Could you check a few things on this model? Use its own coordinates, in mm. Face numbers are marked on the shaded views. A direction names the side the tool comes from. Give positions to 0.01 mm unless a question says otherwise; leave off trailing zeros. Order: outer loops, then holes, each group sorted by start corner. A loop starts at its lowest first (then second) coordinate and runs counter-clockwise, first axis right, second up. Notation, with made-up numbers: (10, 27) -> (15, 27) arc R10 ccw to (15, 34) -> close; hole circle Ø6 at (37.25, 57). An arc over 180 degrees is marked (long way). One line per item, written item: value.
```python
from build123d import *

# Parameters (mm, degrees)
SKETCH1_W           = 55
SKETCH1_H           = 38
SKETCH1_R           = 14.2875
BOSS_EXTRUDE3_DEPTH = 8
SKETCH8_W           = 6
SKETCH8_H           = 38
BOSS_EXTRUDE6_DEPTH = 35
FILLET1_R           = 1
SKETCH9_R           = 2.5
CUT_EXTRUDE1_DEPTH  = 10


with BuildPart() as part:
    # Sketch1 → Boss-Extrude3 (new body)
    with BuildSketch(Plane.XY):
        with Locations((27.5, 19)):
            Rectangle(SKETCH1_W, SKETCH1_H)
        with Locations((35, 19)):
            Circle(SKETCH1_R, mode=Mode.SUBTRACT)
    extrude(amount=BOSS_EXTRUDE3_DEPTH)

    # Sketch8 → Boss-Extrude6 (add)
    with BuildSketch(Plane(origin=(0, 0, 0), x_dir=(-1, 0, 0), z_dir=(0, 0, -1))):
        with Locations((-3, 19)):
            Rectangle(SKETCH8_W, SKETCH8_H)
    extrude(amount=BOSS_EXTRUDE6_DEPTH)

    # Fillet1
    fillet1_edges = [part.edges().sort_by_distance(p)[0] for p in [
        (6, 19, 0),
    ]]
    fillet(fillet1_edges, radius=FILLET1_R)

    # Sketch9 → Cut-Extrude1 (cut)
    with BuildSketch(Plane(origin=(6, 0, 0), x_dir=(0, 0, -1), z_dir=(1, 0, 0))):
        with Locations((8.157894737, 30)):
            Circle(SKETCH9_R)
        with Locations((8.157894737, 8)):
            Circle(SKETCH9_R)
        with Locations((27.842105263, 8)):
            Circle(SKETCH9_R)
        with Locations((27.842105263, 30)):
            Circle(SKETCH9_R)
    extrude(amount=-CUT_EXTRUDE1_DEPTH, mode=Mode.SUBTRACT)


solid = part.part
```
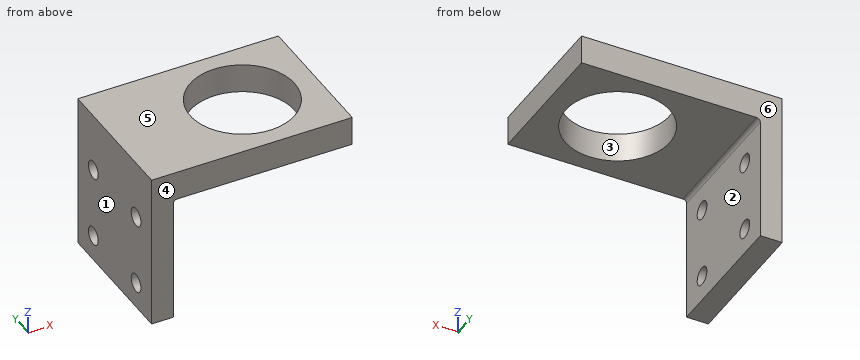
1) If I drill on line 1 along X through (y, z) = (18.5, 4.5); line 2 along Y through (x, z) = (35, 2); line 3 along Z through (x, y) = (52.5, 16), over which ranges is the centre line in solid material (lowest first)?
Answer below:
line 1: x = 0 to 20.72, 49.28 to 55
line 2: y = 0 to 4.71, 33.29 to 38
line 3: z = 0 to 8
2) Suppose I cut it at D-D, the plane y = 3.5. Write out the boundary of the cut face in (x, z).
Answer below:
outline: (0, -35) -> (6, -35) -> (6, -1) arc R1 cw to (7, 0) -> (55, 0) -> (55, 8) -> (0, 8) -> close
3) For P1, Ø2, axis at y = 6.5, z = -27.5, coming from the +X side; P2, Ø6, axis at x = 14.5, y = 19.5, coming from the -Z side; P3, Ø4, axis at y = 30, z = -27.84, coming from the -X side, each with a flat end and sliding along its axis, tell me the tip position at first contact or that it passes through.
Answer below:
P1: stops at x = 6
P2: stops at z = 0
P3: passes through
4) Suppose I cut it at B-B, the plane y = 19. Write out the boundary of the cut face in (x, z).
Answer below:
outline: (0, -35) -> (6, -35) -> (6, -1) arc R1 cw to (7, 0) -> (20.71, 0) -> (20.71, 8) -> (0, 8) -> close; (49.29, 0) -> (55, 0) -> (55, 8) -> (49.29, 8) -> close
5) Suppose I cut it at C-C, the plane x = 4.5. Write out the boundary of the cut face in (y, z), then the cut area to 3 significant figures.
Answer below:
outline: (0, -35) -> (38, -35) -> (38, 8) -> (0, 8) -> close; hole circle Ø5 at (8, -27.84); hole circle Ø5 at (8, -8.16); hole circle Ø5 at (30, -27.84); hole circle Ø5 at (30, -8.16)
area: 1,560 mm2
6) We'd pull the mould along Y, two halves only. Please class the marked faces 3, 4, 5 and 6: +Y half, -Y half, draft (parallel to the pull), parting line (faces both ways), or undercut.
Answer below:
face 3: undercut
face 4: -Y half
face 5: draft
face 6: +Y half
7) Suppose I cut it at A-A, the plane x = 35. Write out the boundary of the cut face in (y, z), then the cut area to 3 significant figures.
Answer below:
outline: (0, 0) -> (4.71, 0) -> (4.71, 8) -> (0, 8) -> close; (33.29, 0) -> (38, 0) -> (38, 8) -> (33.29, 8) -> close
area: 75.4 mm2
8) For the marked faces 1 and 2, which set-ups out of +Z, -Z, +X, -X, +Y, -Y let a thin tool reach every point of the face, with its end or its side?
Answer below:
face 1: +Z, -Z, -X, +Y, -Y
face 2: -Z, +X, +Y, -Y
